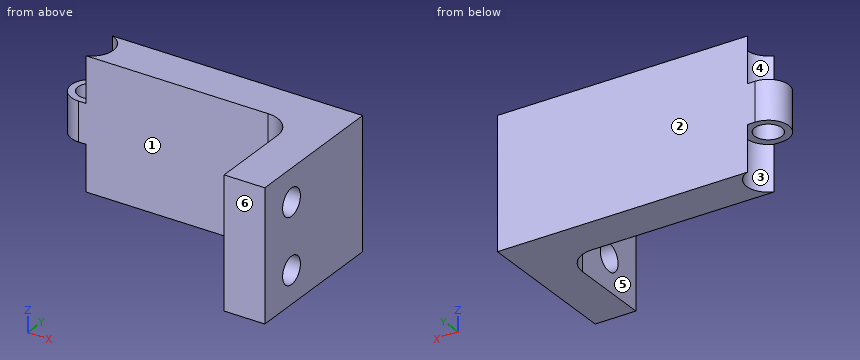
from build123d import *

# Parameters (mm, degrees)
F0_R     = 1.5875
F1_DEPTH = 15.24
F3_W     = 2.54
F3_H     = 5.334
F5_R     = 1.5875
F6_DEPTH = 4.7635


with BuildPart() as f1:
    # F0 (on Top) → F1 (new body)
    with BuildSketch(Plane.XY):
        with BuildLine():
            ThreePointArc((-3.175, 0), (-0.929936, -0.929936), (0, -3.175))
            Line((0, -3.175), (0, -12.7))
            Line((0, -12.7), (4.7625, -12.7))
            Line((4.7625, -12.7), (4.7625, 4.7625))
            Line((4.7625, 4.7625), (-25.4, 4.7625))
            ThreePointArc((-25.4, 4.7625), (-27.78125, 2.38125), (-25.4, 0))
            Line((-25.4, 0), (-3.175, 0))
        make_face()
        with Locations((-25.4, 2.38125)):
            Circle(F0_R, mode=Mode.SUBTRACT)
    extrude(amount=F1_DEPTH)

    # F3 (on offset) → F4 (revolve, cut)
    with BuildSketch(Plane.XZ.offset(-2.38125)):
        with Locations((-26.67, 12.573)):
            Rectangle(F3_W, F3_H)
        with Locations((-26.67, 2.667)):
            Rectangle(F3_W, F3_H)
    revolve(axis=Axis((-25.4, 2.38125, 12.573), (0, 0, -1)), mode=Mode.SUBTRACT)

    # F5 (on face) → F6 (cut, through all)
    with BuildSketch(Plane(origin=(0, 0, 0), x_dir=(0, -1, 0), z_dir=(-1, 0, 0))):
        with Locations((7.9375, 11.43)):
            Circle(F5_R)
        with Locations((7.9375, 3.81)):
            Circle(F5_R)
    extrude(amount=-F6_DEPTH, mode=Mode.SUBTRACT)


solid = f1.part
The model under review builds one solid part; all positions refer to its coordinate system, in mm. Face numbers are marked on the shaded views. A direction names the side the tool comes from. Give positions to 0.01 mm unless a question says otherwise; leave off trailing zeros. Loops run counter-clockwise (first coordinate to the right, second up) from the corner with the lowest first, then second, coordinate; pieces in that order, holes last. Notation, with made-up numbers: (-30, 5.25) -> (19, 5.25) arc R11 cw to (19, 18.25) -> close; hole circle Ø7 at (8, 2.5). An arc over 180 degrees is marked (long way). Put each result on its own line as item: value. Start each with the question number.
1. Wall thickness on probe 1 along Y at (x, z) = (-25.4, 7.1); probe 2 along Y at (x, z) = (3, 11.5); probe 3 along Y at (x, z) = (-19.5, 10.75): over which ranges is each line inside the solid? List them lowest first.
2. We need section C-C on y = -10. State the section outline as (x, z) points, then the cut area to 3 significant figures.
3. For the marked faces 1 and 2, list the 3-axis set-ups (+Z, -Z, +X, -X, +Y, -Y) from which the entire face can be reached by the end or side of a thin tool; tool diameter is ignored.
4. Mouldability with a two-part tool opening along Y and no side actions: class the marked faces 3, 4, 5 and 6 as released by +Y, released by -Y, zero draft, split by the parting line, or undercut.
5. Clearance check with flat-ended pins moving along their axes: P1, Ø8, axis at y = -10.5, z = 7, coming from the -X side; P2, Ø3, axis at x = -25.4, y = 2.38, coming from the +Z side; P3, Ø3, axis at x = -18, z = 5.5, coming from the -Y side; P4, Ø2.5, axis at x = -25, y = 2, coming from the +Z side. State where each tip first meets the part, or that it passes through.
Determined:
1. probe 1: 0 to 0.79, 3.97 to 4.76
1. probe 2: -12.7 to -9.52, -6.35 to 4.76
1. probe 3: 0 to 4.76
2. outline: (0, 0) -> (4.76, 0) -> (4.76, 15.24) -> (0, 15.24) -> close
2. area: 72.6 mm^2
3. face 1: +Z, -Z, -X, -Y
3. face 2: +Z, -Z, +X, -X, +Y
4. face 3: undercut
4. face 4: undercut
4. face 5: zero draft
4. face 6: released by -Y
5. P1: x = 0
5. P2: through
5. P3: y = 0
5. P4: z = 9.91
